Answer from the drawing. Dimensions are ordinates in mm from the lowest x, y and z of the part. Round coordinates to 2 decimals unless told otherwise and drop trailing zeros. Write each loop counter-clockwise with the first axis right and the second up, starting at its lowest first coordinate (ties: lowest second). Pieces come first, ordered by that corner, then holes. Notation, with made-up numbers: M 26,67.25 L 68,67.25 A4 ccw 68,73.25 Z; hole C 66.5,-4.5 d6. An arc over 180 degrees is marked long. One line per item, written item: value. Start each with the question number.
(1) Section A-A (y = 20) is taken. Determine the outline of the cut face in (x, z), plus the area to 3 significant figures.
(2) For a pull along Z with two mould halves and no side action, classify the marked faces 1, 2 and 3 as released by +Z, released by -Z, zero draft, split by the parting line, or undercut.
(3) Section C-C (x = 5.5) is taken. Determine the outline of the cut face in (y, z).
(4) Section D-D (y = 43.5) is taken. Determine the outline of the cut face in (x, z).
(5) Consider probe 1 along Y at (x, z) = (6.35, 6.5); probe 2 along Z at (x, y) = (9.5, 43.5); probe 3 along Y at (x, z) = (6.35, 4.5). Determine where each line is inside the solid, lowest interval first.
(6) Section B-B (z = 7.5) is taken. Determine the outline of the cut face in (x, y).
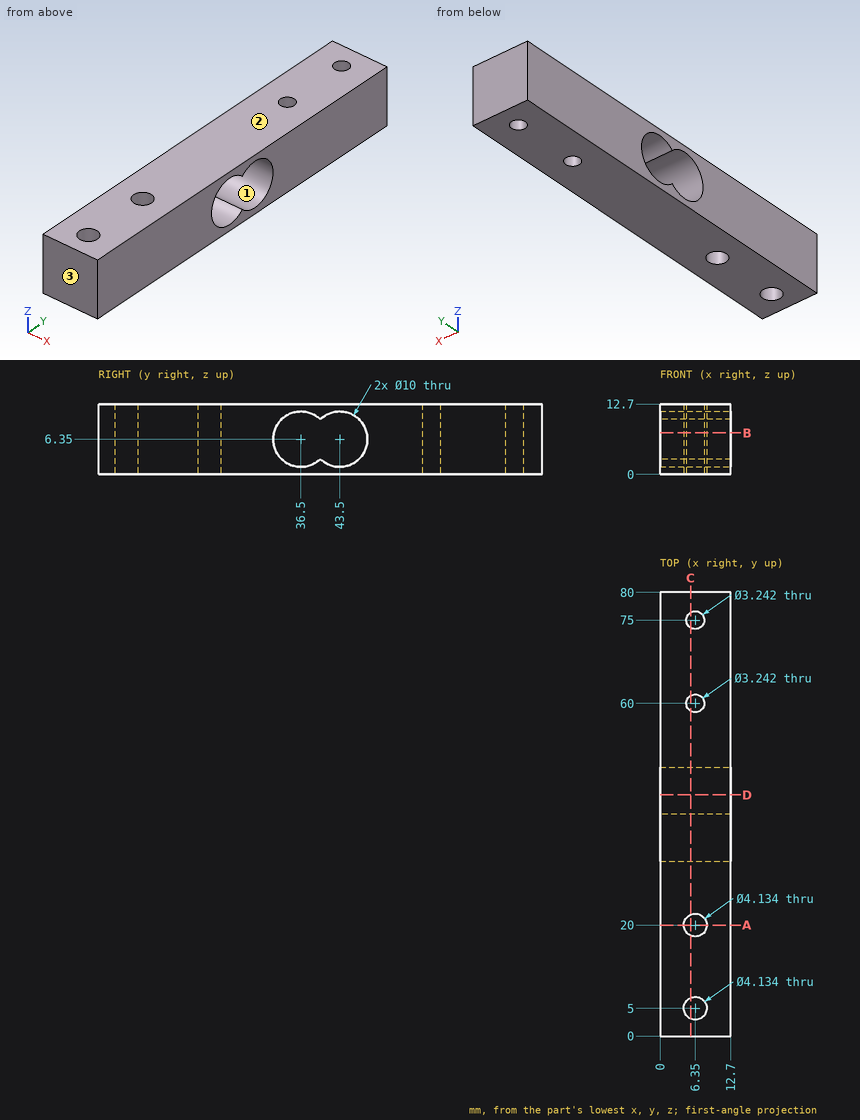
Recorded:
1. outline: M 0,0 L 4.28,0 L 4.28,12.7 L 0,12.7 Z; M 8.42,0 L 12.7,0 L 12.7,12.7 L 8.42,12.7 Z
1. area: 109 mm2
2. face 1: undercut
2. face 2: released by +Z
2. face 3: zero draft
3. outline: M 0,0 L 3.12,0 L 3.12,12.7 L 0,12.7 Z; M 6.88,0 L 18.12,0 L 18.12,12.7 L 6.88,12.7 Z; M 21.88,0 L 58.62,0 L 58.62,12.7 L 21.88,12.7 Z; M 61.38,0 L 73.62,0 L 73.62,12.7 L 61.38,12.7 Z; M 76.38,0 L 80,0 L 80,12.7 L 76.38,12.7 Z; hole M 40,2.78 A5 ccw long 40,9.92 A5 ccw long Z
4. outline: M 0,0 L 12.7,0 L 12.7,1.35 L 0,1.35 Z; M 0,11.35 L 12.7,11.35 L 12.7,12.7 L 0,12.7 Z
5. probe 1: y = 0 to 2.93, 7.07 to 17.93, 22.07 to 31.5, 48.5 to 58.38, 61.62 to 73.38, 76.62 to 80
5. probe 2: z = 0 to 1.35, 11.35 to 12.7
5. probe 3: y = 0 to 2.93, 7.07 to 17.93, 22.07 to 31.85, 48.15 to 58.38, 61.62 to 73.38, 76.62 to 80
6. outline: M 0,0 L 12.7,0 L 12.7,31.63 L 0,31.63 Z; M 0,48.37 L 12.7,48.37 L 12.7,80 L 0,80 Z; hole C 6.35,5 d4.13; hole C 6.35,20 d4.13; hole C 6.35,60 d3.24; hole C 6.35,75 d3.24
